```python
from build123d import *

# Parameters (mm, degrees)
F0_W         = 58.9547399431
F0_H         = 51.2344771996
F0_W_2       = 38.1
F0_H_2       = 38.1
F1_DEPTH     = 57.404
F2_R         = 12.4366404678
F3_DEPTH     = 25.4
F4_W         = 104.0811147541
F4_H         = 122.5580200553
F5_DEPTH     = 25.4
F6_DEPTH     = 25.4
F7_R         = 6.690453714
F8_DEPTH     = 25.4
F9_W         = 129.4811147541
F9_H         = 27.0336512476
F9_W_2       = 264.7406511664
F10_DEPTH    = 142.24
F11_T1_DEPTH = 1466.3511823856
F12_DEPTH    = 251.46
F16_W        = 33.5519401288
F16_H        = 256.0288235545
F17_DEPTH    = 25.4
F19_DEPTH    = 25.4
F20_W        = 66.9628661126
F20_H        = 59.9260473394
F21_DEPTH    = 190.5


# Not quite as in the source:
# - a fillet or chamfer that OpenCascade refuses, or shapes differently, is made with other operations: its cross-section is extruded or revolved along the edge and cut away or added
# - a feature of the source that left no trace in its solid (it failed there, or was rolled back) is left out


with BuildPart() as f1:
    # F0 (on Front) → F1 (new body)
    with BuildSketch(Plane.XZ):
        with Locations((-1.0527623817, -16.6687513702)):
            Rectangle(F0_W, F0_H)
        with Locations((-0.9248415082, -14.9141447619)):
            Rectangle(F0_W_2, F0_H_2, mode=Mode.SUBTRACT)
    extrude(amount=F1_DEPTH)

    # F2 (on face) → F3 (cut)
    with BuildSketch(Plane(origin=(-30.5301323533, 0, 0), x_dir=(0, -1, 0), z_dir=(-1, 0, 0))):
        with Locations((28.702, -17.1130020171)):
            Circle(F2_R)
    extrude(amount=-F3_DEPTH, mode=Mode.SUBTRACT)

    # F4 (on face) → F5 (join)
    with BuildSketch(Plane(origin=(0, 0, 0), x_dir=(-1, 0, 0), z_dir=(0, 1, 0))):
        with Locations((22.4943133071, -18.3081142604)):
            Rectangle(F4_W, F4_H)
    extrude(amount=F5_DEPTH)

    # F6 (add): a face of the model
    f6_faces = [f1.faces().sort_by_distance(p)[0] for p in [
        (-74.5348706841, 12.7, -18.3081142604),
    ]]
    extrude(f6_faces, amount=F6_DEPTH)

    # F7 (on face) → F8 (cut)
    with BuildSketch(Plane(origin=(-30.5301323533, 0, 0), x_dir=(0, -1, 0), z_dir=(-1, 0, 0))):
        with Locations((8.7604233995, -30.5925961584)):
            Circle(F7_R)
    extrude(amount=-F8_DEPTH, mode=Mode.SUBTRACT)

    # F9 (on face) → F10 (join)
    with BuildSketch(Plane(origin=(0, 25.4, 0), x_dir=(-1, 0, 0), z_dir=(0, 1, 0))):
        with Locations((35.1943133071, 29.4540701434)):
            Rectangle(F9_W, F9_H)
        with Locations((232.3051962674, 29.4540701434)):
            Rectangle(F9_W_2, F9_H)
    extrude(amount=F10_DEPTH)

    # F11: fillet of radius 362.4072547021 on 1 edges, made by hand

    # F11_s2 → F11_t1 (cut)
    with BuildSketch(Plane.XY.offset(-703.7215210494)):
        with BuildLine():
            ThreePointArc((-76.812015623, 167.64), (-237.3561028838, 130.139830949), (-364.6755218506, 25.4))
            Line((-364.6755218506, 25.4), (-364.6755218506, 167.64))
            Line((-364.6755218506, 167.64), (-76.812015623, 167.64))
        make_face()
    extrude(amount=F11_T1_DEPTH, mode=Mode.SUBTRACT)

    # F12 (add): a face of the model
    f12_faces = [f1.faces().sort_by_distance(p)[0] for p in [
        (-99.9348706841, 12.7, -18.3081142604),
    ]]
    extrude(f12_faces, amount=F12_DEPTH)

    # F15: F1 across face


with BuildPart() as f1_1:
    add(f1.part)
    add(f1.part.mirror(Plane(origin=(-160.9243133071, 12.7, -79.5871242881), x_dir=(1, 0, 0), z_dir=(0, 0, -1))))

    # F16 (on face) → F17 (join)
    with BuildSketch(Plane.XZ):
        with Locations((-334.6189006197, -74.1307325661)):
            Rectangle(F16_W, F16_H)
    extrude(amount=F17_DEPTH)

    # F18 (on face) → F19 (cut)
    with BuildSketch(Plane.XZ):
        Polygon((-295.2485382557, -116.8882586062), (-295.2485382557, -170.68554461), (-30.5301323533, -170.68554461), (-30.5301323533, -168.1227358058), (-30.5301323533, -116.8882586062), align=None)
        Polygon((-296.9728708267, 8.9484872296), (-296.9728708267, -47.0983237028), (-18.4958036989, -47.0983237028), (-18.4958036989, -42.28598997), (-30.5301323533, -42.28598997), (-30.5301323533, 8.9484872296), align=None)
    extrude(amount=-F19_DEPTH, mode=Mode.SUBTRACT)

    # F20 (on face) → F21 (join)
    with BuildSketch(Plane(origin=(0, 0, 15.9372445196), x_dir=(1, 0, 0), z_dir=(0, 0, -1))):
        with Locations((-3.9351889864, -137.6769763303)):
            Rectangle(F20_W, F20_H)
    extrude(amount=F21_DEPTH)


solid = f1_1.part
```
The listing builds one solid part. Answer for the finished solid, in the listing's coordinates (mm). A direction names the side the tool comes from. Round coordinates to 2 decimals unless told otherwise and drop trailing zeros. Write each loop counter-clockwise with the first axis right and the second up, starting at its lowest first coordinate (ties: lowest second). Pieces come first, ordered by that corner, then holes. Notation, with made-up numbers: (-5, 15.25) -> (32, 15.25) arc R25 cw to (32, 50.25) -> close; hole circle Ø8 at (-1.75, -13). An arc over 180 degrees is marked (long way). Use CSV: the item, a comma, the result in double quotes. Start each with the question number.
(1) Section C-C on x = -237.5 is taken. Give the vertices of the cut face in (y, z), then the cut area to 3 significant figures.
(2) Consider L1, parallel to Z at x = -161, y = 85.5; L2, parallel to Y at x = -296.5, z = -102.5; L3, parallel to X at y = 5, z = 17. Determine where each line is inside the solid, lowest interval first. Write a range as from..to.
(3) Section B-B on y = 116 is taken. Give the vertices of the cut face in (x, z), then the cut area to 3 significant figures.
(4) Each of these flat-tipped pins is pushed along its axis until it touches: pin 1 (3 mm diameter, centred on x = -50.5, y = 8.5, fed in from +Z); pin 2 (3.5 mm diameter, centred on x = -335, z = 48, fed in from +Y); pin 3 (10 mm diameter, centred on y = 22.5, z = -139.5, fed in from -X). Where does it stop, or does it pass through?
(5) Which of the six approach directions +Z, -Z, +X, -X, +Y, -Y give full straight-line access (tool end or side, diameter ignored) to faces 5 (the face through (-1, -28, -168.123)), 6 (the face through (28.425, -28, -142)), 7 (the face through (-1, -28, -125.21))?
(6) Section D-D on x = -94 is taken. Give the vertices of the cut face in (y, z).
(7) The mould has two halves that part along X. Classify faces 1 (the face through (-165, 80, 15.937)), 2 (the face through (-296.973, 13, -19)), 3 (the face through (18.125, -28, -144)), 4 (the face through (28.425, -28, -17)): released by +X, released by -X, zero draft, split by the parting line, or undercut.
(8) Section A-A on z = -96 is taken. Give the vertices of the cut face in (x, y).
A:
1,outline,"(0, -202.15) -> (130.07, -202.15) -> (130.07, -175.11) -> (25.4, -175.11) -> (25.4, -170.69) -> (0, -170.69) -> close; (0, -116.89) -> (25.4, -116.89) -> (25.4, -47.1) -> (0, -47.1) -> close; (0, 8.95) -> (25.4, 8.95) -> (25.4, 15.94) -> (130.07, 15.94) -> (130.07, 42.97) -> (0, 42.97) -> close"
1,area,"9,100 mm²"
2,L1,"z = -202.15..-175.11, 15.94..42.97"
2,L2,"y = 0..25.4"
2,L3,"x = -351.39..29.55"
3,outline,"(-263.26, -202.15) -> (29.55, -202.15) -> (29.55, -175.11) -> (-263.26, -175.11) -> close; (-263.26, 15.94) -> (-37.42, 15.94) -> (-37.42, -174.56) -> (29.55, -174.56) -> (29.55, 42.97) -> (-263.26, 42.97) -> close"
3,area,"28,600 mm²"
4,pin 1,"stops at z = 42.97"
4,pin 2,"stops at y = 0"
4,pin 3,"stops at x = -351.39"
5,face 5,"-Z, +X, -Y"
5,face 6,"+Z, -Z, +X, -Y"
5,face 7,"-Y"
6,outline,"(0, -202.15) -> (167.23, -202.15) -> (167.23, -175.11) -> (25.4, -175.11) -> (25.4, -170.69) -> (0, -170.69) -> close; (0, -116.89) -> (25.4, -116.89) -> (25.4, -47.1) -> (0, -47.1) -> close; (0, 8.95) -> (25.4, 8.95) -> (25.4, 15.94) -> (167.23, 15.94) -> (167.23, 42.97) -> (0, 42.97) -> close"
7,face 1,"zero draft"
7,face 2,"undercut"
7,face 3,"undercut"
7,face 4,"released by +X"
8,outline,"(-351.39, -25.4) -> (-317.84, -25.4) -> (-317.84, 0) -> (29.55, 0) -> (29.55, 25.4) -> (-351.39, 25.4) -> close; (-37.42, 107.71) -> (29.55, 107.71) -> (29.55, 167.64) -> (-37.42, 167.64) -> close"
